```python
from build123d import *

# Parameters (mm, degrees)
F0_W     = 120
F0_H     = 120
F1_DEPTH = 30
F2_R     = 35
F3_DEPTH = 25
F4_R     = 25
F5_DEPTH = 55.001
F6_R     = 5
F7_R     = 1.5
F8_T     = -2


with BuildPart() as f1:
    # F0 (on Front) → F1 (new body)
    with BuildSketch(Plane.XZ):
        Rectangle(F0_W, F0_H)
    extrude(amount=F1_DEPTH)

    # F2 (on face) → F3 (join)
    with BuildSketch(Plane.XZ.offset(30)):
        Circle(F2_R)
    extrude(amount=F3_DEPTH)

    # F4 (on face) → F5 (cut, through all)
    with BuildSketch(Plane.XZ.offset(55)):
        Circle(F4_R)
    extrude(amount=-F5_DEPTH, mode=Mode.SUBTRACT)

    # F6
    f6_edges = [f1.edges().sort_by_distance(p)[0] for p in [
        (-35, -30, 0),
        (0, -30, 60),
        (60, -30, 0),
        (60, -15, 60),
        (60, -15, -60),
        (0, -30, -60),
        (-60, -15, -60),
        (-60, -30, 0),
        (-60, -15, 60),
    ]]
    fillet(f6_edges, radius=F6_R)

    # F7
    f7_edges = [f1.edges().sort_by_distance(p)[0] for p in [
        (-35, -55, 0),
    ]]
    fillet(f7_edges, radius=F7_R)

    # F8
    f8_openings = [f1.faces().sort_by_distance(p)[0] for p in [
        (58.302944, 0, 0),
    ]]
    offset(amount=F8_T, openings=f8_openings)


solid = f1.part
```
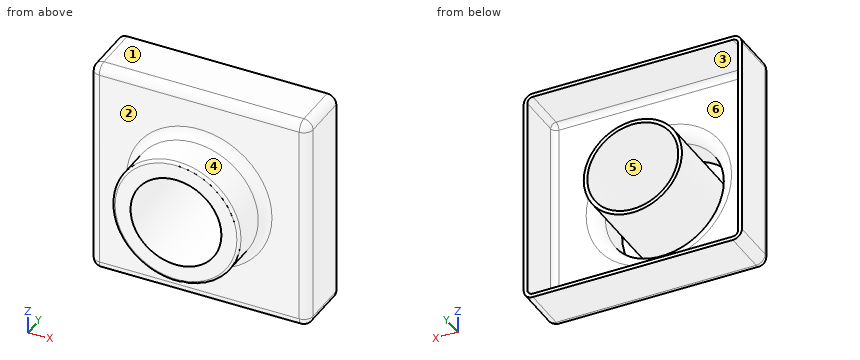
For this review, take the finished solid that the model builds, in its own axes (mm). Face numbers are marked on the shaded views. A direction names the side the tool comes from. Round coordinates to 2 decimals unless told otherwise and drop trailing zeros. Write each loop counter-clockwise with the first axis right and the second up, starting at its lowest first coordinate (ties: lowest second). Pieces come first, ordered by that corner, then holes. Notation, with made-up numbers: (-33.5, -32.5) -> (20.5, -32.5) arc R11 ccw to (20.5, -24.5) -> close; hole circle Ø4 at (-37, 20.5). An arc over 180 degrees is marked (long way). One line per question, with ' | ' between items. Start each with the question number.
(1) Add section D-D, the plane z = -47. Write out the cut boundary in (x, y).
(2) For line 1 along Z through (x, y) = (0, -42); line 2 along X through (y, z) = (-24, -33); line 3 along X through (y, z) = (-48, 22), list the stretches that pass through material, from the lowest coordinate up. Write a range as from..to.
(3) Insertion check: P1, Ø6, axis at y = -29.5, z = -4, coming from the +X side; P2, Ø6, axis at x = 0, y = -40.5, coming from the -Z side; P3, Ø1.5, axis at y = -28.5, z = -7, coming from the +X side. Each pin has a flat end and moves straight along its axis. Give the tip position at first contact, or say it passes through.
(4) Mouldability with a two-part tool opening along Z and no side actions: class the marked faces 1, 2 and 3 as released by +Z, released by -Z, zero draft, split by the parting line, or undercut.
(5) Tool access review of the marked faces 4, 5 and 6: name each direction out of +Z, -Z, +X, -X, +Y, -Y from which nothing blocks a thin tool from reaching the whole face with its end or side.
(6) Add section A-A, the plane y = -3. Write out the cut boundary in (x, z).
Answer list:
1) outline: (-60, -25) arc R5 ccw to (-55, -30) -> (55, -30) arc R5 ccw to (60, -25) -> (60, 0) -> (58, 0) -> (58, -25) arc R3 cw to (55, -28) -> (-55, -28) arc R3 cw to (-58, -25) -> (-58, 0) -> (-60, 0) -> close
2) line 1: -35..-33, -27..-25, 25..27, 33..35 | line 2: -60..-58, 58..60 | line 3: -27.22..-24.6, -15.65..-11.87, 11.87..15.65, 24.6..27.22
3) P1: x = 59.77 | P2: z = -35 | P3: x = 59.18
4) face 1: released by +Z | face 2: zero draft | face 3: undercut
5) face 4: -Y | face 5: +Y, -Y | face 6: +Y
6) outline: (-60, -55) arc R5 ccw to (-55, -60) -> (55, -60) arc R5 ccw to (60, -55) -> (60, 55) arc R5 ccw to (55, 60) -> (-55, 60) arc R5 ccw to (-60, 55) -> close; circle Ø54 at (0, 0); hole (-58, -55) arc R3 ccw to (-55, -58) -> (55, -58) arc R3 ccw to (58, -55) -> (58, 55) arc R3 ccw to (55, 58) -> (-55, 58) arc R3 ccw to (-58, 55) -> close; hole circle Ø50 at (0, 0)
